Drawing for the job (mm, zero at the part's lowest x, y, z). A direction names the side the tool comes from. Coordinates: 2 decimals unless noted, no trailing zeros. Order: outer loops, then holes, each group sorted by start corner. A loop starts at its lowest first (then second) coordinate and runs counter-clockwise, first axis right, second up. Notation, with made-up numbers: (56, 23.25) - (62, 23.25) arc R28 ccw to (62, 59.25) - close; hole circle Ø2 at (64.5, 49). An arc over 180 degrees is marked (long way). Put each result on its own line as item: value. Start each with the question number.
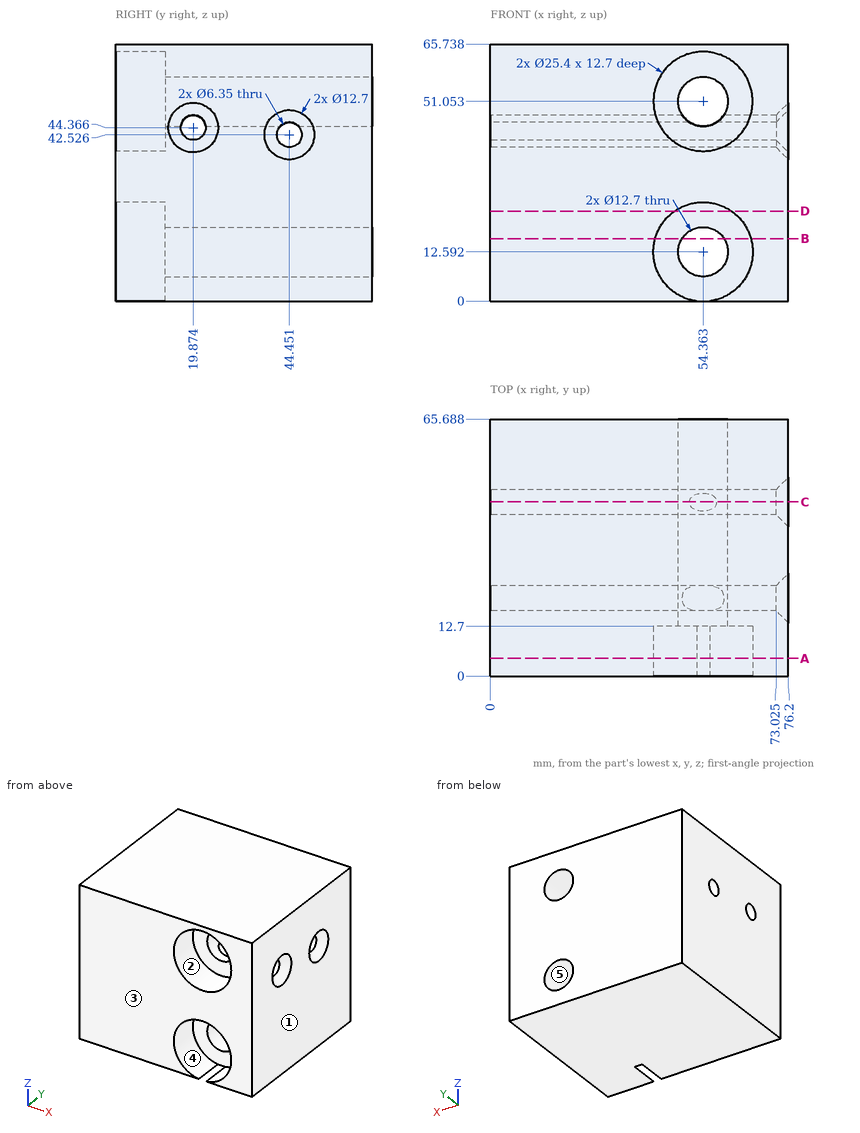
Item 1: 3-axis set-ups, long thin cutter, end or side, ignore diameter. For the marked faces 4 and 5: which of +Z, -Z, +X, -X, +Y, -Y reach the whole face in a straight line?
Item 2: Slice it at C-C, the plane y = 44.5. Give the number of separate pieces and of enclosed holes in the cut face, plus the area to 3 significant figures.
Item 3: Slice it at A-A, the plane y = 4.5. Give the cut face in (x, z), plus the area to 3 significant figures.
Item 4: Wall check: line 1 along Z through (x, y) = (54, 26); line 2 along Z through (x, y) = (58.5, 3.5) (1 decimal); line 3 along Y through (x, z) = (50, 56). Give the ranges that are in metal, low to high.
Item 5: Slice it at B-B, the plane z = 16. Give the cut face in (x, y) (1 decimal), plus the area to 3 significant figures.
Item 6: Flat gauge pin, fed straight in: pin 1 Ø20.5 at (x, z) = (54.36, 51.05) entering from -Y. Where does the tip first touch, or does it go through?
Item 7: Slice it at D-D, the plane z = 23. Give the cut face in (x, y).
Item 8: Pull direction X, two halves, no side cores. Call the marked faces 1, 2 and 3: pulls with the +X half, pulls with the -X half, needs draft (parallel to the pull), parting line crosses it, or undercut.
Here are the results:
1. face 4: -Y
1. face 5: +Y, -Y
2. separate pieces: 2
2. enclosed holes: 1
2. area: 4,270 mm^2
3. outline: (0, 0) - (52.71, 0) arc R12.7 cw (long way) to (56.02, 0) - (76.2, 0) - (76.2, 65.74) - (0, 65.74) - close; hole circle Ø25.4 at (54.36, 51.05)
3. area: 4,000 mm^2
4. line 1: z = 0 to 6.25, 18.93 to 44.71, 57.39 to 65.74
4. line 2: z = 0 to 0.6, 24.6 to 39, 63.1 to 65.7
4. line 3: y = 12.7 to 65.69
5. outline: (0, 0) - (42.1, 0) - (42.1, 12.7) - (49, 12.7) - (49, 65.7) - (0, 65.7) - close; (59.7, 12.7) - (66.6, 12.7) - (66.6, 0) - (76.2, 0) - (76.2, 65.7) - (59.7, 65.7) - close
5. area: 4,130 mm^2
6. pin 1: stops at y = 12.7
7. outline: (0, 0) - (47.09, 0) - (47.09, 12.7) - (61.64, 12.7) - (61.64, 0) - (76.2, 0) - (76.2, 65.69) - (0, 65.69) - close
8. face 1: pulls with the +X half
8. face 2: undercut
8. face 3: needs draft
